Here's how the part is built. I have some questions about the finished solid (model axes, mm). Face numbers are marked on the shaded views. A direction names the side the tool comes from. Give positions to 0.01 mm unless a question says otherwise; leave off trailing zeros. Loops run counter-clockwise (first coordinate to the right, second up) from the corner with the lowest first, then second, coordinate; pieces in that order, holes last. Notation, with made-up numbers: (49.25, 51.5) - (102.25, 51.5) arc R24 ccw to (102.25, 76.5) - close; hole circle Ø3 at (57, -8.75). An arc over 180 degrees is marked (long way). Use one line per item in the form item = value.
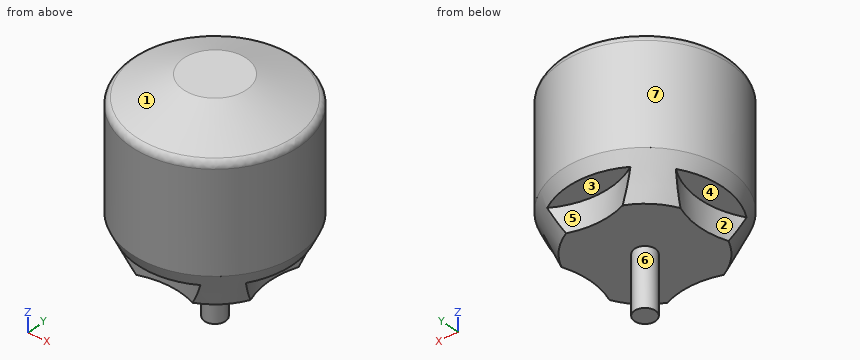
from build123d import *

# Parameters (mm, degrees)
F0_R     = 32
F1_DEPTH = 64
F2_SIZE2 = 9
F2_SIZE  = 20
F3_SIZE2 = 7
F3_SIZE  = 15
F4_R     = 3
F5_R     = 30
F7_DEPTH = 10
F6_R     = 4
F8_DEPTH = 22


with BuildPart() as f1:
    # F0 (on Top) → F1 (new body)
    with BuildSketch(Plane.XY):
        Circle(F0_R)
    extrude(amount=F1_DEPTH)

    # F2
    f2_edges = [f1.edges().sort_by_distance(p)[0] for p in [
        (-32, 0, 64),
    ]]
    f2_side = f1.faces().sort_by_distance((0, 0, 64))[0]
    chamfer(f2_edges, length=F2_SIZE, length2=F2_SIZE2, reference=f2_side)

    # F3
    f3_edges = [f1.edges().sort_by_distance(p)[0] for p in [
        (-32, 0, 0),
    ]]
    f3_side = f1.faces().sort_by_distance((-32, 0, 27.5))[0]
    chamfer(f3_edges, length=F3_SIZE, length2=F3_SIZE2, reference=f3_side)

    # F4
    f4_edges = [f1.edges().sort_by_distance(p)[0] for p in [
        (-32, 0, 55),
    ]]
    fillet(f4_edges, radius=F4_R)

    # F5 (on face) → F7 (cut)
    with BuildSketch(Plane(origin=(0, 0, 0), x_dir=(1, 0, 0), z_dir=(0, 0, -1))):
        with Locations((-50.605738163, 0)):
            Circle(F5_R)
        with Locations((0, -50.605738163)):
            Circle(F5_R)
        with Locations((50.605738163, 0)):
            Circle(F5_R)
        with Locations((0, 50.605738163)):
            Circle(F5_R)
    extrude(amount=-F7_DEPTH, mode=Mode.SUBTRACT)

    # F6 (on face) → F8 (join)
    with BuildSketch(Plane(origin=(0, 0, 0), x_dir=(1, 0, 0), z_dir=(0, 0, -1))):
        Circle(F6_R)
    extrude(amount=F8_DEPTH)


solid = f1.part
(1) If we section it at B-B (z = -8): List the corners of the cut face in (x, y) for me, plus the area to 3 significant figures.
Geometry says:
outline = circle Ø8 at (0, 0)
area = 50.3 mm²
(2) If we section it at C-C (z = 41): List the corners of the cut face in (x, y) for me, plus the area to 3 significant figures.
Geometry says:
outline = circle Ø64 at (0, 0)
area = 3,220 mm²
(3) For P1, Ø8, axis at x = -2.5, z = 9.5, coming from the -Y side; P2, Ø1.5, axis at x = 16, y = 4.5, coming from the +Z side; P3, Ø10, axis at x = 21.5, y = -23, coming from the -Z side, each with a flat end and sliding along its axis, tell me the tip position at first contact or that it passes through.
Geometry says:
P1 = -31.22
P2 = 62.26
P3 = 3.18
(4) If I drill on probe 1 along Y at (x, z) = (1, 38.5); probe 2 along X at (y, z) = (12, 36); probe 3 along Z at (x, y) = (-18, -9), over which ranges is the centre line in solid material (lowest first)?
Geometry says:
probe_1 = -31.98 to 31.98
probe_2 = -29.66 to 29.66
probe_3 = 0 to 60.34
(5) For the marked faces 4, 5, 6 and 7, which set-ups out of +Z, -Z, +X, -X, +Y, -Y let a thin tool reach every point of the face, with its end or its side?
Geometry says:
face_4 = -Z, -X
face_5 = -Z, +Y
face_6 = -Z
face_7 = +Z, -Z
(6) If we section it at A-A (z = 7.5): List the corners of the cut face in (x, y) for me, plus the area to 3 significant figures.
Geometry says:
outline = (-24.44, -14.67) arc R28.5 ccw to (-14.67, -24.44) arc R30 cw to (14.67, -24.44) arc R28.5 ccw to (24.44, -14.67) arc R30 cw to (24.44, 14.67) arc R28.5 ccw to (14.67, 24.44) arc R30 cw to (-14.67, 24.44) arc R28.5 ccw to (-24.44, 14.67) arc R30 cw to start
area = 1,930 mm²
(7) Thinking about a two-plate mould opening in X: for the marked faces 1, 2 and 3, which applies, pulls with the +X half, pulls with the -X half, needs draft (parallel to the pull), parting line crosses it, or undercut?
Geometry says:
face_1 = parting line crosses it
face_2 = pulls with the -X half
face_3 = undercut
